Model file for the job. Use its own axes, mm. A direction names the side the tool comes from. Coordinates: 2 decimals unless noted, no trailing zeros. Order: outer loops, then holes, each group sorted by start corner. A loop starts at its lowest first (then second) coordinate and runs counter-clockwise, first axis right, second up.
from build123d import *


with BuildPart() as f1:
    # F0 (on Front) → F1 (revolve)
    with BuildSketch(Plane.XZ):
        Polygon((-42.576, 32.322101), (0, 32.322101), (0, 75.121), (-72.891891, 75.121), (-72.891891, 60.854718), (-62.192168, 60.854718), (-62.192168, 51.938277), (-51.938262, 51.938277), (-51.938262, 42.130191), (-42.576, 42.130191), align=None)
        Polygon((0, 75.121), (0, 32.322101), (42.576, 32.322101), (42.576, 42.130191), (51.938262, 42.130191), (51.938262, 51.938277), (62.192168, 51.938277), (62.192168, 60.854718), (72.891891, 60.854718), (72.891891, 75.121), align=None)
    revolve(axis=Axis((0.891461, 0, 0), (1, 0, 0)))


solid = f1.part
Q1. Mould opens along Y. For faces 1 (the face through (42.576, 31, 10)), 2 (the face through (-72.892, 61, -6)), 3 (the face through (-1.02, 45.71, -59.613)) say: pulls with the +Y half, pulls with the -Y half, needs draft (parallel to the pull), parting line crosses it, or undercut.
Established:
face 1: undercut
face 2: needs draft
face 3: parting line crosses it
Q2. Probe line 1 (Z direction, x = -65, y = 0); line 2 (Y direction, x = -49, z = 0); line 3 (Z direction, x = 6.5, y = 1). List the from-to ranges inside material, lowest first.
Established:
line 1: z = -75.12 to -60.85, 60.85 to 75.12
line 2: y = -75.12 to -42.13, 42.13 to 75.12
line 3: z = -75.11 to -32.31, 32.31 to 75.11
Q3. Cut at C-C, the plane x = 21.5. List the corners of the cut face in (y, z).
Established:
outline: circle Ø150.24 at (0, 0); hole circle Ø64.64 at (0, 0)
Q4. Which spindle directions (+Z, -Z, +X, -X, +Y, -Y) get a long thin tool onto all of the face, cutting with end or side? Do faces 4 (the face through (67.617, -2.676, -60.796)), 5 (the face through (-51.938, -43, 0)), 6 (the face through (72.892, 61, 6)). Say none if no direction does.
Established:
face 4: +X
face 5: -X
face 6: +Z, -Z, +X, +Y, -Y
Q5. Cut at D-D, the plane z = -44.5. List the corners of the cut face in (x, y).
Established:
outline: (-72.89, -60.52) - (72.89, -60.52) - (72.89, -41.51) - (62.19, -41.51) - (62.19, -26.78) - (51.94, -26.78) - (51.94, 26.78) - (62.19, 26.78) - (62.19, 41.51) - (72.89, 41.51) - (72.89, 60.52) - (-72.89, 60.52) - (-72.89, 41.51) - (-62.19, 41.51) - (-62.19, 26.78) - (-51.94, 26.78) - (-51.94, -26.78) - (-62.19, -26.78) - (-62.19, -41.51) - (-72.89, -41.51) - close
Q6. Drop flat-ended pins along their axis: P1, Ø6, axis at x = 48.5, y = -43.5, coming from the +Z side; P2, Ø2, axis at x = -48.5, z = -43, coming from the +Y side; P3, Ø1.5, axis at x = -15.5, y = -57, coming from the +Z side; P4, Ø12, axis at y = -18, z = -17, coming from the +X side. Give the stop position or say it passes through.
Established:
P1: stops at z = 63.27
P2: stops at y = 62.28
P3: stops at z = 49.79
P4: passes through
